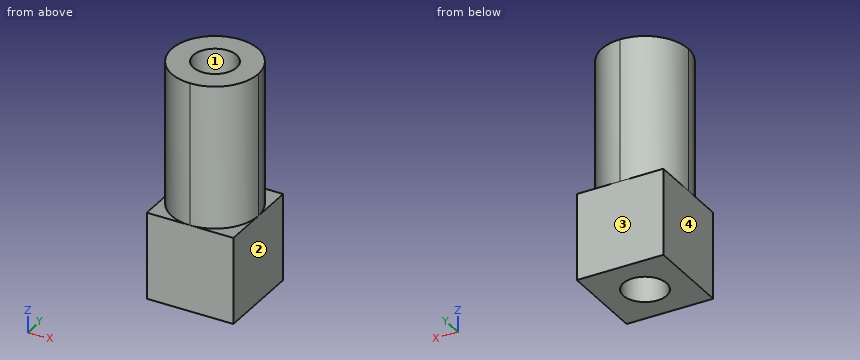
from build123d import *

# Parameters (mm, degrees)
F0_W     = 50.8
F0_H     = 50.8
F1_DEPTH = 50.8
F3_DEPTH = 83.82
F4_R     = 12.7
F5_DEPTH = 143.764


with BuildPart() as f1:
    # F0 (on Top) → F1 (new body)
    with BuildSketch(Plane.XY):
        with Locations((-25.4, 25.4)):
            Rectangle(F0_W, F0_H)
    extrude(amount=-F1_DEPTH)

    # F2 (on face) → F3 (join)
    with BuildSketch(Plane.XY):
        with BuildLine():
            ThreePointArc((-25.4, 0), (-7.439488, 7.439488), (0, 25.4))
            ThreePointArc((0, 25.4), (-7.439488, 43.360512), (-25.4, 50.8))
            ThreePointArc((-25.4, 50.8), (-43.360512, 43.360512), (-50.8, 25.4))
            ThreePointArc((-50.8, 25.4), (-43.360512, 7.439488), (-25.4, 0))
        make_face()
    extrude(amount=F3_DEPTH)

    # F4 (on face) → F5 (cut)
    with BuildSketch(Plane.XY.offset(83.82)):
        with Locations((-25.4, 25.4)):
            Circle(F4_R)
    extrude(amount=-F5_DEPTH, mode=Mode.SUBTRACT)


solid = f1.part
Can you work these out from the model? Positions are in its coordinate system, mm. Face numbers are marked on the shaded views. Give positions to 0.01 mm unless a question says otherwise; leave off trailing zeros. Write each loop counter-clockwise with the first axis right and the second up, starting at its lowest first coordinate (ties: lowest second). Pieces come first, ordered by that corner, then holes. Notation, with made-up numbers: (-36, -10.5) -> (21, -10.5) arc R18 ccw to (21, 17.5) -> close; hole circle Ø5 at (-29, 51). An arc over 180 degrees is marked (long way). Answer as a JSON object with one key per item and string values. Group by question number.
Item 1: Suppose I cut it at A-A (x = -21.5). Please give me the cut outline in (y, z), plus the area to 3 significant figures.
Item 2: I'm going to push flat-ended pins straight in: P1, Ø1.5, axis at y = 40.5, z = 70, coming from the +X side; P2, Ø1, axis at x = -7, y = 44.5, coming from the +Z side; P3, Ø5, axis at x = -9.5, z = 55.5, coming from the +Y side. Where does each tip first touch, or does it pass through?
Item 3: Suppose I cut it at B-B (z = 40.5). Please give me the cut outline in (x, y).
Item 4: Suppose I cut it at C-C (y = 34.5). Please give me the cut outline in (x, z).
Item 5: Please list where these lines run through material, in increasing order: line 1 (Y direction, x = -25.4, z = -19); line 2 (X direction, y = 25, z = 30); line 3 (X direction, y = 20, z = -16.5). Write a range as [from, to].
Item 6: Suppose I cut it at D-D (x = -10). Please give me the cut outline in (y, z), plus the area to 3 significant figures.
Item 7: We'd pull the mould along X, two halves only. Please class the marked faces 1, 2, 3 and 4: +X half, -X half, draft (parallel to the pull), parting line (faces both ways), or undercut.
Findings:
{
 "1": {"outline": "(0, -50.8) -> (13.31, -50.8) -> (13.31, 83.82) -> (0.3, 83.82) -> (0.3, 0) -> (0, 0) -> close; (37.49, -50.8) -> (50.8, -50.8) -> (50.8, 0) -> (50.5, 0) -> (50.5, 83.82) -> (37.49, 83.82) -> close", "area": "3,530 mm²"},
 "2": {"P1": "stops at x = -4.44", "P2": "stops at z = 0", "P3": "stops at y = 46.98"},
 "3": {"outline": "(-50.8, 25.4) arc R25.4 ccw to (-25.4, 0) arc R25.4 ccw to (0, 25.4) arc R25.4 ccw to (-25.4, 50.8) arc R25.4 ccw to start; hole circle Ø25.4 at (-25.4, 25.4)"},
 "4": {"outline": "(-50.8, -50.8) -> (-34.26, -50.8) -> (-34.26, 83.82) -> (-49.11, 83.82) -> (-49.11, 0) -> (-50.8, 0) -> close; (-16.54, -50.8) -> (0, -50.8) -> (0, 0) -> (-1.69, 0) -> (-1.69, 83.82) -> (-16.54, 83.82) -> close"},
 "5": {"line 1": "y = [0, 12.7], [38.1, 50.8]", "line 2": "x = [-50.8, -38.09], [-12.71, 0]", "line 3": "x = [-50.8, -36.89], [-13.91, 0]"},
 "6": {"outline": "(0, -50.8) -> (50.8, -50.8) -> (50.8, 0) -> (45.6, 0) -> (45.6, 83.82) -> (5.2, 83.82) -> (5.2, 0) -> (0, 0) -> close", "area": "5,970 mm²"},
 "7": {"face 1": "undercut", "face 2": "+X half", "face 3": "draft", "face 4": "-X half"}
}
